from build123d import *

# Parameters (mm, degrees)
F1_DEPTH = 10
F3_D     = 1.5
F4_R     = 2


with BuildPart() as f1:
    # F0 (on Top) → F1 (new body)
    with BuildSketch(Plane.XY):
        with BuildLine():
            ThreePointArc((-6, 0), (0, 6), (6, 0))
            Line((6, 0), (6, -3))
            Line((6, -3), (18, -3))
            Line((18, -3), (18, 0))
            Line((18, 0), (9, 0))
            ThreePointArc((9, 0), (0, 9), (-9, 0))
            Line((-9, 0), (-18, 0))
            Line((-18, 0), (-18, -3))
            Line((-18, -3), (-6, -3))
            Line((-6, -3), (-6, 0))
        make_face()
    extrude(amount=F1_DEPTH)

    # F3 (through all)
    with Locations(Plane(origin=(0, 0, 0), x_dir=(-1, 0, 0), z_dir=(0, 1, 0))):
        with Locations((-13.5, 5), (13.5, 5)):
            Hole(F3_D / 2)

    # F4
    f4_edges = [f1.edges().sort_by_distance(p)[0] for p in [
        (9, 0, 5),
        (-9, 0, 5),
    ]]
    fillet(f4_edges, radius=F4_R)


solid = f1.part
Can you work these out from the model? Positions are in its coordinate system, mm. A direction names the side the tool comes from. Coordinates: 2 decimals unless noted, no trailing zeros. Loops run counter-clockwise (first coordinate to the right, second up) from the corner with the lowest first, then second, coordinate; pieces in that order, holes last. Notation, with made-up numbers: (74.5, -29.75) - (105.5, -29.75) arc R23 cw to (105.5, -18.75) - close; hole circle Ø1 at (47, 29.25). An arc over 180 degrees is marked (long way). Put each result on its own line as item: value. Start each with the question number.
Item 1: Which directions (+Z, -Z, +X, -X, +Y, -Y) give clear straight access to the entire face, cutting with the end or side of a thin tool? Please do faces 5 (the face through (-6, -2, 5)), 6 (the face through (9.55, 0.45, 5.07)), 7 (the face through (-14.4, 0, 4.9)).
Item 2: If we mould it in two halves opening along X, with no side actions, what happens to faces 1 (the face through (12.75, -1.52, 5.03)), 2 (the face through (-18, -1, 5)), 3 (the face through (-14.25, -1.52, 5.03)), 4 (the face through (14.5, 0, 4.9))? For each: +X half, -X half, draft (parallel to the pull), parting line (faces both ways), or undercut.
Item 3: Suppose I cut it at C-C (x = 13.5). Please give me the cut outline in (y, z), and give its area (3 significant figures).
Item 4: Suppose I cut it at A-A (y = -1.25). Please give me the cut outline in (x, z), and give its area (3 significant figures).
Item 5: Suppose I cut it at D-D (y = 4.25). Please give me the cut outline in (x, z), and give its area (3 significant figures).
Item 6: If I drill on line 1 along Z through (x, y) = (-13.5, -1.2); line 2 along X through (y, z) = (5.25, 5.5); line 3 along X through (y, z) = (1.5, 3.25), over which ranges is the centre line in solid material (lowest first)?
Item 7: For pin 1 (2 mm diameter, centred on y = 4.5, z = 7.5, fed in from -X); pin 2 (3 mm diameter, centred on y = 2, z = 1, fed in from +X); pin 3 (1.5 mm diameter, centred on y = 2.5, z = 1.5, fed in from +X); pin 4 (1.7 mm diameter, centred on x = -13.5, z = 5, fed in from -Y), each with a flat end and sliding along its axis, tell me the tip position at first contact or that it passes through.
Item 8: Suppose I cut it at B-B (z = 5). Please give me the cut outline in (x, y), and give its area (3 significant figures).
Here are the results:
1. face 5: +Z, -Z, -Y
1. face 6: +Z, -Z, +X, +Y
1. face 7: +Z, -Z, -X, +Y
2. face 1: undercut
2. face 2: -X half
2. face 3: undercut
2. face 4: draft
3. outline: (-3, 0) - (0, 0) - (0, 4.25) - (-3, 4.25) - close; (-3, 5.75) - (0, 5.75) - (0, 10) - (-3, 10) - close
3. area: 25.5 mm²
4. outline: (-18, 0) - (-6, 0) - (-6, 10) - (-18, 10) - close; (6, 0) - (18, 0) - (18, 10) - (6, 10) - close; hole circle Ø1.5 at (-13.5, 5); hole circle Ø1.5 at (13.5, 5)
4. area: 236 mm²
5. outline: (-7.93, 0) - (-4.24, 0) - (-4.24, 10) - (-7.93, 10) - close; (4.24, 0) - (7.93, 0) - (7.93, 10) - (4.24, 10) - close
5. area: 74.0 mm²
6. line 1: 0 to 4.25, 5.75 to 10
6. line 2: -7.31 to -2.9, 2.9 to 7.31
6. line 3: -8.88 to -5.81, 5.81 to 8.88
7. pin 1: x = -8.29
7. pin 2: x = 9.49
7. pin 3: x = 8.83
7. pin 4: y = -3
8. outline: (-18, -3) - (-14.25, -3) - (-14.25, 0) - (-18, 0) - close; (-12.75, -3) - (-6, -3) - (-6, 0) arc R6 cw to (6, 0) - (6, -3) - (12.75, -3) - (12.75, 0) - (10.82, 0) arc R2 cw to (8.85, 1.64) arc R9 ccw to (-8.85, 1.64) arc R2 cw to (-10.82, 0) - (-12.75, 0) - close; (14.25, -3) - (18, -3) - (18, 0) - (14.25, 0) - close
8. area: 135 mm²
